The listing builds one solid part. Answer for the finished solid, in the listing's coordinates (mm). Coordinates: 2 decimals unless noted, no trailing zeros. Order: outer loops, then holes, each group sorted by start corner. A loop starts at its lowest first (then second) coordinate and runs counter-clockwise, first axis right, second up. Notation, with made-up numbers: (62, -24) - (119, -24) arc R17 cw to (119, -5) - close; hole circle Ø7 at (59, 72.5). An arc over 180 degrees is marked (long way). One line per item, written item: value. Start each with the question number.
```python
from build123d import *

# Parameters (mm, degrees)
SKETCH1_W               = 20.32
SKETCH1_H               = 20.32
SKETCH1_R               = 4.765
BOSS_EXTRUDE1_DEPTH     = 20.32
CUT_EXTRUDE1_DEPTH      = 18.597636205
CUT_EXTRUDE1_DEPTH_BACK = 18.597636205
SKETCH2_R               = 4.765


with BuildPart() as part:
    # Sketch1 → Boss-Extrude1 (new body)
    with BuildSketch(Plane.XY):
        Rectangle(SKETCH1_W, SKETCH1_H)
        Circle(SKETCH1_R, mode=Mode.SUBTRACT)
    extrude(amount=BOSS_EXTRUDE1_DEPTH)

    # Sketch2 → Cut-Extrude1 (cut, two sides: drawn at the far end of the back side and taken through both)
    with BuildSketch(Plane(origin=(0, 0, 10.16), x_dir=(0, 0, -1), z_dir=(1, 0, 0)).offset(-CUT_EXTRUDE1_DEPTH_BACK)):
        Circle(SKETCH2_R)
    extrude(amount=CUT_EXTRUDE1_DEPTH + CUT_EXTRUDE1_DEPTH_BACK, mode=Mode.SUBTRACT)


solid = part.part
```
(1) A flat-ended cylindrical pin translates along its axis: pin 1 Ø8.5 at (y, z) = (0, 10.16) entering from +X. Find the tip coordinate at first contact, or state that the pin passes through.
(2) The part is cut by section D-D on x = 3.25. Determine the outline of the cut face in (y, z) (3 decimals), plus the area to 3 significant figures.
(3) Consider probe 1 along Z at (x, y) = (-6, 0) (3 decimals); probe 2 along X at (y, z) = (0, 15.5) (3 decimals); probe 3 along Y at (x, z) = (-0.25, 12.5). Determine where each line is inside the solid, lowest interval first.
(4) For a pull along Y with two mould halves and no side action, classify faces 1 (the face through (0, -10.16, 10)), 2 (the face through (6.14, 0.21, 14.92)), 3 (the face through (10.16, -5, 8)) as pulls with the +Y half, pulls with the -Y half, needs draft (parallel to the pull), parting line crosses it, or undercut.
(5) The part is cut by section A-A on y = 0. Determine the outline of the cut face in (x, z) (3 decimals), plus the area to 3 significant figures.
(6) The part is cut by section B-B on z = 17. Determine the outline of the cut face in (x, y) (3 decimals).
(7) The part is cut by section C-C on x = -8.5. Determine the outline of the cut face in (y, z) (3 decimals), plus the area to 3 significant figures.
Completed:
1. pin 1: passes through
2. outline: (-10.16, 0) - (-3.485, 0) - (-3.485, 6.91) arc R4.765 cw to (-3.485, 13.41) - (-3.485, 20.32) - (-10.16, 20.32) - close; (3.485, 0) - (10.16, 0) - (10.16, 20.32) - (3.485, 20.32) - (3.485, 13.41) arc R4.765 cw to (3.485, 6.91) - close
2. area: 260 mm2
3. probe 1: z = 0 to 5.395, 14.925 to 20.32
3. probe 2: x = -10.16 to -4.765, 4.765 to 10.16
3. probe 3: y = -10.16 to -4.76, 4.76 to 10.16
4. face 1: pulls with the -Y half
4. face 2: undercut
4. face 3: needs draft
5. outline: (-10.16, 0) - (-4.765, 0) - (-4.765, 5.395) - (-10.16, 5.395) - close; (-10.16, 14.925) - (-4.765, 14.925) - (-4.765, 20.32) - (-10.16, 20.32) - close; (4.765, 0) - (10.16, 0) - (10.16, 5.395) - (4.765, 5.395) - close; (4.765, 14.925) - (10.16, 14.925) - (10.16, 20.32) - (4.765, 20.32) - close
5. area: 116 mm2
6. outline: (-10.16, -10.16) - (10.16, -10.16) - (10.16, 10.16) - (-10.16, 10.16) - close; hole circle Ø9.53 at (0, 0)
7. outline: (-10.16, 0) - (10.16, 0) - (10.16, 20.32) - (-10.16, 20.32) - close; hole circle Ø9.53 at (0, 10.16)
7. area: 342 mm2
